Answer from the drawing. Dimensions are ordinates in mm from the lowest x, y and z of the part. A direction names the side the tool comes from. Give positions to 0.01 mm unless a question says otherwise; leave off trailing zeros. Write each loop counter-clockwise with the first axis right and the second up, starting at its lowest first coordinate (ties: lowest second). Pieces come first, ordered by that corner, then holes. Notation, with made-up numbers: (-40, -12.75) -> (-30, -12.75) arc R5 cw to (-30, -5.75) -> close; hole circle Ø10 at (-20.5, -13.5). An arc over 180 degrees is marked (long way). Put each result on its own line as item: value. Start each with the question number.
1) For a pull along X with two mould halves and no side action, classify the marked faces 1, 2 and 3 as released by +X, released by -X, zero draft, split by the parting line, or undercut.
2) A cutting plane is placed at A-A (y = 74.5). Write down the section's boundary in (x, z), then the cut area to 3 significant figures.
3) A cutting plane is placed at D-D (z = 92.5). Write down the section's boundary in (x, y), then the cut area to 3 significant figures.
4) For the marked faces 4, 5 and 6, determine the directions among +Z, -Z, +X, -X, +Y, -Y from which every point of the face is accessible in a straight line to the end or side of a thin tool.
5) A cutting plane is placed at B-B (x = 747.5). Write down the section's boundary in (y, z).
6) A cutting plane is placed at C-C (z = 370.5). Write down the section's boundary in (x, y).
7) Find the intervals of material crossed by line 1 along X through (y, z) = (18, 374); line 2 along Z through (x, y) = (836, 95); line 3 along Y through (x, z) = (740, 279.5), in increasing order. Write a range as from..to.
8) Flat-ended cylindrical pins translate along their axes: pin 1 Ø1.5 at (y, z) = (132, 183) entering from -X; pin 2 Ø8 at (x, z) = (695.5, 171) entering from -Y; pin 3 Ø6 at (x, y) = (532, 95) entering from -Z. Find the tip coordinate at first contact, or state that the pin passes through.
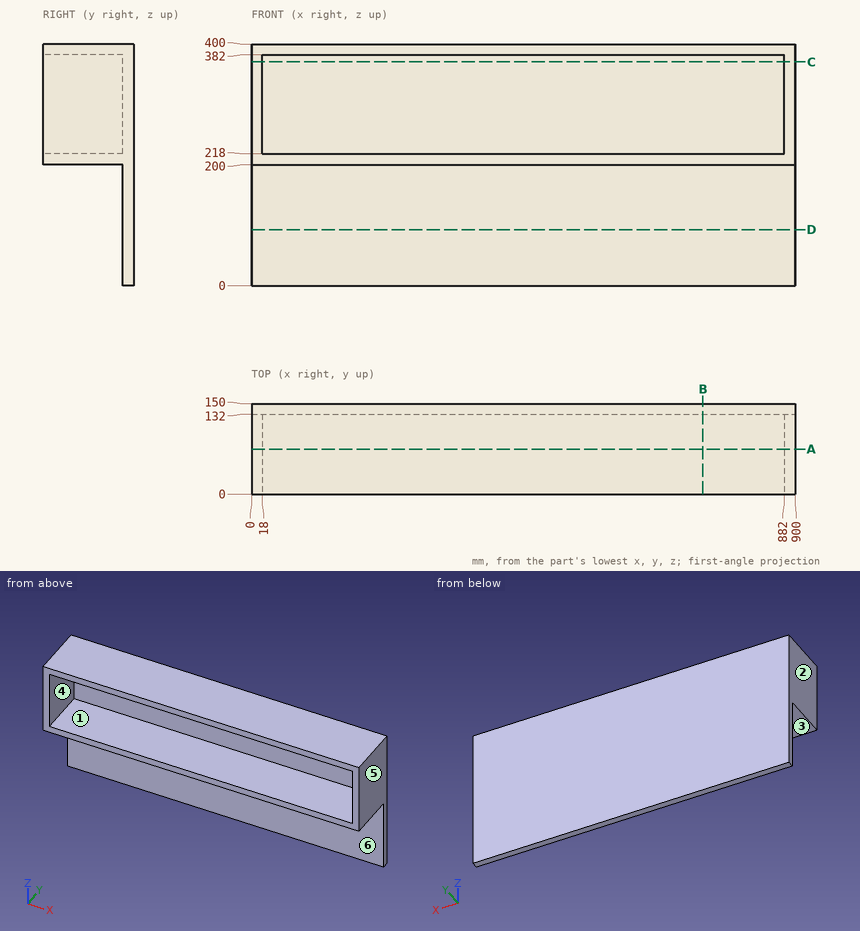
Reply:
1. face 1: undercut
1. face 2: released by -X
1. face 3: zero draft
2. outline: (0, 200) -> (900, 200) -> (900, 400) -> (0, 400) -> close; hole (18, 218) -> (882, 218) -> (882, 382) -> (18, 382) -> close
2. area: 38,300 mm2
3. outline: (0, 132) -> (900, 132) -> (900, 150) -> (0, 150) -> close
3. area: 16,200 mm2
4. face 4: -Y
4. face 5: +Z, -Z, +X, +Y, -Y
4. face 6: -Z, +X, -X, -Y
5. outline: (0, 200) -> (132, 200) -> (132, 0) -> (150, 0) -> (150, 400) -> (0, 400) -> (0, 382) -> (132, 382) -> (132, 218) -> (0, 218) -> close
6. outline: (0, 0) -> (18, 0) -> (18, 132) -> (882, 132) -> (882, 0) -> (900, 0) -> (900, 150) -> (0, 150) -> close
7. line 1: x = 0..18, 882..900
7. line 2: z = 200..218, 382..400
7. line 3: y = 132..150
8. pin 1: stops at x = 0
8. pin 2: stops at y = 132
8. pin 3: stops at z = 200
